Study the drawing (mm; zero at the part's minimum x, y, z) and answer. A direction names the side the tool comes from. Round coordinates to 2 decimals unless told otherwise and drop trailing zeros. Loops run counter-clockwise (first coordinate to the right, second up) from the corner with the lowest first, then second, coordinate; pieces in that order, holes last. Notation, with made-up numbers: (48, -14) -> (93, -14) arc R20 ccw to (93, 13) -> close; hole circle Ø10 at (60, -6.5). An arc over 180 degrees is marked (long way). Write each question's results on one line, items separated by ' | '. Start each with the question number.
(1) Straight lines are drawn through the part: probe 1 along Y at (x, z) = (7.48, 11.25); probe 2 along Y at (x, z) = (7.48, 5.75); probe 3 along Z at (x, y) = (7, 36). For each, find the intervals that lie inside material, in ascending order.
(2) A flat-ended cylindrical pin translates along its axis: pin 1 (6 mm diameter, centred on x = 2, y = 23.5, fed in from -Z). Find the tip coordinate at first contact, or state that the pin passes through.
(3) The part is cut by section B-B (x = 13.75). Determine the outline of the cut face in (y, z).
(4) For the marked faces 4 and 5, determine the directions among +Z, -Z, +X, -X, +Y, -Y from which every point of the face is accessible in a straight line to the end or side of a thin tool.
(5) The part is cut by section A-A (x = 7.48). Determine the outline of the cut face in (y, z).
(6) Determine the mould class of the marked faces 1, 2 and 3 for opening direction X: released by +X, released by -X, zero draft, split by the parting line, or undercut.
(7) The part is cut by section C-C (z = 11.46). Determine the outline of the cut face in (x, y), plus the area to 3 significant figures.
(8) The part is cut by section D-D (y = 6). Determine the outline of the cut face in (x, z), plus the area to 3 significant figures.
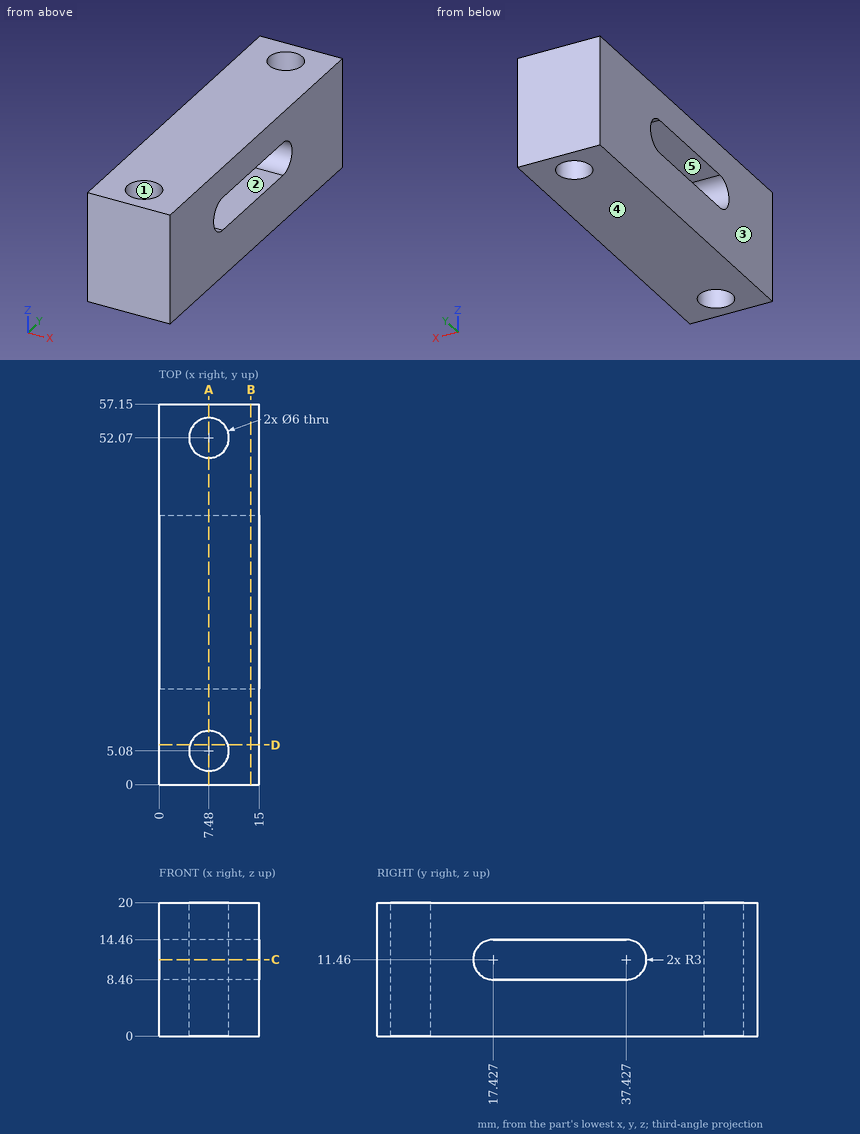
Checked values:
1) probe 1: y = 0 to 2.08, 8.08 to 14.43, 40.42 to 49.07, 55.07 to 57.15 | probe 2: y = 0 to 2.08, 8.08 to 49.07, 55.07 to 57.15 | probe 3: z = 0 to 8.46, 14.46 to 20
2) pin 1: stops at z = 0
3) outline: (0, 0) -> (57.15, 0) -> (57.15, 20) -> (0, 20) -> close; hole (17.43, 8.46) -> (37.43, 8.46) arc R3 ccw to (37.43, 14.46) -> (17.43, 14.46) arc R3 ccw to start
4) face 4: -Z, +X, -X, +Y, -Y | face 5: +X, -X
5) outline: (0, 0) -> (2.08, 0) -> (2.08, 20) -> (0, 20) -> close; (8.08, 0) -> (49.07, 0) -> (49.07, 20) -> (8.08, 20) -> close; (55.07, 0) -> (57.15, 0) -> (57.15, 20) -> (55.07, 20) -> close; hole (17.43, 8.46) -> (37.43, 8.46) arc R3 ccw to (37.43, 14.46) -> (17.43, 14.46) arc R3 ccw to start
6) face 1: undercut | face 2: zero draft | face 3: released by -X
7) outline: (0, 0) -> (15, 0) -> (15, 14.43) -> (0, 14.43) -> close; (0, 40.43) -> (15, 40.43) -> (15, 57.15) -> (0, 57.15) -> close; hole circle Ø6 at (7.48, 5.08); hole circle Ø6 at (7.48, 52.07) | area: 411 mm2
8) outline: (0, 0) -> (4.62, 0) -> (4.62, 20) -> (0, 20) -> close; (10.34, 0) -> (15, 0) -> (15, 20) -> (10.34, 20) -> close | area: 186 mm2
